from build123d import *

# Parameters (mm, degrees)
SKETCH1_R           = 30
SKETCH1_R_2         = 20
BOSS_EXTRUDE1_DEPTH = 60
BOSS_EXTRUDE3_START = -15
SKETCH2_R           = 10
BOSS_EXTRUDE3_DEPTH = 15
BOSS_EXTRUDE4_START = -30
BOSS_EXTRUDE4_DEPTH = 15
BOSS_EXTRUDE8_DEPTH = 30
SKETCH9_R           = 8
CUT_EXTRUDE2_DEPTH  = 22.929058222
BOSS_EXTRUDE9_START = 45
BOSS_EXTRUDE9_DEPTH = 45
CUT_EXTRUDE8_DEPTH  = 10


with BuildPart() as part:
    # Sketch1 → Boss-Extrude1 (new body)
    with BuildSketch(Plane.XY):
        Circle(SKETCH1_R)
        Circle(SKETCH1_R_2, mode=Mode.SUBTRACT)
    extrude(amount=BOSS_EXTRUDE1_DEPTH)

    # Sketch2 → Boss-Extrude3 (add)
    with BuildSketch(Plane.XY.offset(60).offset(BOSS_EXTRUDE3_START)):
        with BuildLine():
            Line((75, 23), (19.261360284, 23))
            ThreePointArc((19.261360284, 23), (27.18309041, 12.691713664), (30, 0))
            ThreePointArc((30, 0), (27.18309041, -12.691713664), (19.261360284, -23))
            Line((19.261360284, -23), (75, -23))
            ThreePointArc((75, -23), (98, 0), (75, 23))
        make_face()
        with Locations((75, 0)):
            Circle(SKETCH2_R, mode=Mode.SUBTRACT)
    extrude(amount=BOSS_EXTRUDE3_DEPTH)

    # Sketch3 → Boss-Extrude4 (add)
    with BuildSketch(Plane.XY.offset(60).offset(BOSS_EXTRUDE4_START)):
        with BuildLine():
            Line((0, -30), (-75, -30))
            Line((-75, -30), (-75, 30))
            Line((-75, 30), (0, 30))
            ThreePointArc((0, 30), (-30, 0), (0, -30))
        make_face()
    extrude(amount=BOSS_EXTRUDE4_DEPTH)

    # Sketch5 → Boss-Extrude8 (add)
    with BuildSketch(Plane(origin=(0, 0, 0), x_dir=(-1, 0, 0), z_dir=(0, 0, -1))):
        with BuildLine():
            Line((75, 5), (75, 30))
            Line((75, 30), (52.070941778, 30))
            Line((52.070941778, 30), (52.070941778, 5))
            Line((52.070941778, 5), (29.580398915, 5))
            ThreePointArc((29.580398915, 5), (29.894915684, 2.508787808), (30, 0))
            ThreePointArc((30, 0), (29.894915684, -2.508787808), (29.580398915, -5))
            Line((29.580398915, -5), (52.070941778, -5))
            Line((52.070941778, -5), (52.070941778, -30))
            Line((52.070941778, -30), (75, -30))
            Line((75, -30), (75, -5))
            Line((75, -5), (75, -4.926312307))
            Line((75, -4.926312307), (75, 4.981002017))
            Line((75, 4.981002017), (75, 5))
        make_face()
    extrude(amount=-BOSS_EXTRUDE8_DEPTH)

    # Sketch9 → Cut-Extrude2 (cut)
    with BuildSketch(Plane.ZY.offset(75)):
        with Locations(Location((15, -17.5, 0), (0, 0, 270))):
            Circle(SKETCH9_R)
        with Locations(Location((15, 17.5, 0), (0, 0, 90))):
            Circle(SKETCH9_R)
    extrude(amount=-CUT_EXTRUDE2_DEPTH, mode=Mode.SUBTRACT)

    # Sketch10 → Boss-Extrude9 (add)
    with BuildSketch(Plane(origin=(0, 0, 45), x_dir=(-1, 0, 0), z_dir=(0, 0, -1)).offset(BOSS_EXTRUDE9_START)):
        with BuildLine():
            Line((-29.580398915, 5), (-54.580398915, 5))
            Line((-54.580398915, 5), (-54.580398915, -5))
            Line((-54.580398915, -5), (-29.580398915, -5))
            ThreePointArc((-29.580398915, -5), (-30, 0), (-29.580398915, 5))
        make_face()
    extrude(amount=-BOSS_EXTRUDE9_DEPTH)

    # Sketch11 → Cut-Extrude8 (cut)
    with BuildSketch(Plane(origin=(0, 5, 0), x_dir=(1, 0, 0), z_dir=(0, 1, 0))):
        Polygon((29.580398915, 0), (54.580398915, -45), (54.580398915, 0), align=None)
    extrude(amount=-CUT_EXTRUDE8_DEPTH, mode=Mode.SUBTRACT)


solid = part.part
Source: CAD feature listing. Evaluate the final solid. Frame: model axes, mm. A direction names the side the tool comes from. Round coordinates to 2 decimals unless told otherwise and drop trailing zeros. Order: outer loops, then holes, each group sorted by start corner. A loop starts at its lowest first (then second) coordinate and runs counter-clockwise, first axis right, second up. Notation, with made-up numbers: (-29.75, 79.5) - (-7.75, 79.5) arc R27 ccw to (-7.75, 114.5) - close; hole circle Ø6 at (26, 39). An arc over 180 degrees is marked (long way). Use a Markdown table: item, result. Add a question column.
1. Section query B-B (z = 19). Return the cut outline in (x, y), then the cut area to 3 significant figures.
2. Section query C-C (x = 13). Return the cut outline in (y, z).
3. First-contact query: pin 1 (1 mm diameter, centred on x = 23, z = 17, fed in from +Y); pin 2 (12 mm diameter, centred on y = 2, z = 21, fed in from +X); pin 3 (6.5 mm diameter, centred on x = -41.5, z = 16.5, fed in from -Y). Flat tips, straight axial feed; report the tip coordinate or a pass-through.
4. Mould query, pull axis Y, two halves, no side actions, for faces 1 (the cylindrical face through (-63.696, 9.508, 14.648)), 2 (the flat face through (41.905, 0.07, 22.185)), 3 (the flat face through (-45, -30, 32)). Classes: +Y half, -Y half, draft (parallel to the pull), parting line (faces both ways), or undercut.
5. Set-up query: faces 4 (the flat face through (48, 23, 52)), 5 (the cylindrical face through (-63.696, -11.151, 10.132)), 6 (the flat face through (37, -5, 32)), 7 (the flat face through (-52.071, -9, 15)). Return all of +Z, -Z, +X, -X, +Y, -Y with unobstructed straight access to the full face (end or side cutting, diameter ignored); none if empty.
6. Section query A-A (y = 0). Return the cut outline in (x, z).
7. Section query D-D (z = 10.5). Return the cut outline in (x, y).
8. Line query: probe 1 along Z at (x, y) = (-58, -17.5); probe 2 along Y at (x, z) = (75, 49); probe 3 along X at (y, z) = (10, 28). Output: solid intervals per line, ascending.
Derived:
| question | item | result |
|---|---|---|
| 1 | outline | (-75, -30) - (-52.07, -30) - (-52.07, -24.43) - (-75, -24.43) - close; (-75, -10.57) - (-52.07, -10.57) - (-52.07, -5) - (-29.58, -5) arc R30 ccw to (29.58, -5) - (40.14, -5) - (40.14, 5) - (29.58, 5) arc R30 ccw to (-29.58, 5) - (-52.07, 5) - (-52.07, 10.57) - (-75, 10.57) - close; (-75, 24.43) - (-52.07, 24.43) - (-52.07, 30) - (-75, 30) - close; hole circle Ø40 at (0, 0) |
| 1 | area | 2,640 mm2 |
| 2 | outline | (-27.04, 0) - (-15.2, 0) - (-15.2, 60) - (-27.04, 60) - close; (15.2, 0) - (27.04, 0) - (27.04, 60) - (15.2, 60) - close |
| 3 | pin 1 | y = 19.84 |
| 3 | pin 2 | x = 44.58 |
| 3 | pin 3 | y = -5 |
| 4 | face 1 | undercut |
| 4 | face 2 | draft |
| 4 | face 3 | -Y half |
| 5 | face 4 | +Z, -Z, +X, +Y |
| 5 | face 5 | -X |
| 5 | face 6 | -Z, +X, -Y |
| 5 | face 7 | -Z, -Y |
| 6 | outline | (-75, 0) - (-20, 0) - (-20, 60) - (-30, 60) - (-30, 45) - (-75, 45) - close; (20, 0) - (29.58, 0) - (54.58, 45) - (65, 45) - (65, 60) - (20, 60) - close; (85, 45) - (98, 45) - (98, 60) - (85, 60) - close |
| 7 | outline | (-75, -30) - (-52.07, -30) - (-52.07, -24.11) - (-75, -24.11) - close; (-75, -10.89) - (-52.07, -10.89) - (-52.07, -5) - (-29.58, -5) arc R30 ccw to (29.58, -5) - (35.41, -5) - (35.41, 5) - (29.58, 5) arc R30 ccw to (-29.58, 5) - (-52.07, 5) - (-52.07, 10.89) - (-75, 10.89) - close; (-75, 24.11) - (-52.07, 24.11) - (-52.07, 30) - (-75, 30) - close; hole circle Ø40 at (0, 0) |
| 8 | probe 1 | 0 to 7, 23 to 45 |
| 8 | probe 2 | -23 to -10, 10 to 23 |
| 8 | probe 3 | -75 to -52.07, -28.28 to -17.32, 17.32 to 28.28 |
